Geometry check sheet. Reference: the model listing, model coordinates, mm. A direction names the side the tool comes from. Round coordinates to 2 decimals unless told otherwise and drop trailing zeros. Write each loop counter-clockwise with the first axis right and the second up, starting at its lowest first coordinate (ties: lowest second). Pieces come first, ordered by that corner, then holes. Notation, with made-up numbers: (8, -26.5) -> (16, -26.5) arc R35 cw to (16, 11.5) -> close; hole circle Ø5 at (-4.5, -17). An arc over 180 degrees is marked (long way). Use a Markdown table: item, result.
```python
from build123d import *

# Parameters (mm, degrees)
SKETCH1_R           = 4
BOSS_EXTRUDE1_DEPTH = 18.288
SKETCH2_R           = 2.625
BOSS_EXTRUDE2_DEPTH = 0.8
SKETCH3_R           = 2
BOSS_EXTRUDE3_DEPTH = 2.4


with BuildPart() as part:
    # Sketch1 → Boss-Extrude1 (new body)
    with BuildSketch(Plane(origin=(0, 0, 0), x_dir=(1, 0, 0), z_dir=(0, 1, 0))):
        Circle(SKETCH1_R)
    extrude(amount=BOSS_EXTRUDE1_DEPTH)

    # Sketch2 → Boss-Extrude2 (add)
    with BuildSketch(Plane(origin=(0, 18.288, 0), x_dir=(1, 0, 0), z_dir=(0, 1, 0))):
        Circle(SKETCH2_R)
    extrude(amount=BOSS_EXTRUDE2_DEPTH)

    # Sketch3 → Boss-Extrude3 (add)
    with BuildSketch(Plane(origin=(0, 19.088, 0), x_dir=(1, 0, 0), z_dir=(0, 1, 0))):
        Circle(SKETCH3_R)
    extrude(amount=BOSS_EXTRUDE3_DEPTH)


solid = part.part
```
(1) Access from +Z, -Z, +X, -X, +Y, -Y to the whole of each face (thin tool, end or side, straight path). Record for faces 1 (the face through (0, 0, 0)), 2 (the face through (3, 18.288, 1)).
A:
| item | result |
|---|---|
| face 1 | +Z, -Z, +X, -X, -Y |
| face 2 | +Y |
(2) Section check D-D on z = -2.25. Record the cut outline in (x, y), plus the area to 3 significant figures.
A:
| item | result |
|---|---|
| outline | (-3.31, 0) -> (3.31, 0) -> (3.31, 18.29) -> (1.35, 18.29) -> (1.35, 19.09) -> (-1.35, 19.09) -> (-1.35, 18.29) -> (-3.31, 18.29) -> close |
| area | 123 mm2 |
(3) Section check C-C on y = 16.5. Record the cut outline in (x, z).
A:
| item | result |
|---|---|
| outline | circle Ø8 at (0, 0) |
(4) Gauge pin test, flat ends, axial feed: pin 1 Ø2 at (y, z) = (10, -3) entering from -X; pin 2 Ø3 at (x, z) = (1, 3) entering from +Y. Record the tip position at first contact, or that the pin passes through.
A:
| item | result |
|---|---|
| pin 1 | stops at x = -3.46 |
| pin 2 | stops at y = 21.49 |
(5) Section check B-B on x = 0. Record the cut outline in (y, z) (3 decimals), plus the area to 3 significant figures.
A:
| item | result |
|---|---|
| outline | (0, -4) -> (18.288, -4) -> (18.288, -2.625) -> (19.088, -2.625) -> (19.088, -2) -> (21.488, -2) -> (21.488, 2) -> (19.088, 2) -> (19.088, 2.625) -> (18.288, 2.625) -> (18.288, 4) -> (0, 4) -> close |
| area | 160 mm2 |
(6) Section check A-A on z = 0. Record the cut outline in (x, y) (3 decimals).
A:
| item | result |
|---|---|
| outline | (-4, 0) -> (4, 0) -> (4, 18.288) -> (2.625, 18.288) -> (2.625, 19.088) -> (2, 19.088) -> (2, 21.488) -> (-2, 21.488) -> (-2, 19.088) -> (-2.625, 19.088) -> (-2.625, 18.288) -> (-4, 18.288) -> close |
(7) Thickness scan on line 1 (Y direction, x = 1.5, z = 2.75); line 2 (Y direction, x = 2, z = -1.25); line 3 (X direction, y = 5.5, z = -1). Record the ranges inside material, lowest first.
A:
| item | result |
|---|---|
| line 1 | y = 0 to 18.29 |
| line 2 | y = 0 to 19.09 |
| line 3 | x = -3.87 to 3.87 |
